```python
from build123d import *

# Parameters (mm, degrees)
BOSS_EXTRUDE1_DEPTH = 0.254
SKETCH2_R           = 4.699
CUT_EXTRUDE1_DEPTH  = 1.254
SKETCH3_W           = 2.54
SKETCH3_H           = 0.635
CUT_EXTRUDE2_DEPTH  = 1.254
SKETCH5_OUTSIDE_W   = 121.447
SKETCH5_OUTSIDE_H   = 109.618
CUT_EXTRUDE5_DEPTH  = 1.254


with BuildPart() as part:
    # Sketch1 → Boss-Extrude1 (new body)
    with BuildSketch(Plane.XY):
        with BuildLine():
            Line((67.21146711, 76.191723231), (8.696654013, 17.676910134))
            Line((8.696654013, 17.676910134), (7.228954972, 14.133571205))
            ThreePointArc((7.228954972, 14.133571205), (14.666587579, 6.075099489), (15.105587123, -4.88230096))
            Line((15.105587123, -4.88230096), (18.648926052, -6.35))
            Line((18.648926052, -6.35), (101.401368334, -6.35))
            ThreePointArc((101.401368334, -6.35), (93.866160503, 38.880636728), (67.21146711, 76.191723231))
        make_face()
        with BuildLine():
            Line((88.672924278, 6.35), (27.86051193, 6.35))
            ThreePointArc((27.86051193, 6.35), (26.399857642, 10.93517908), (24.190484974, 15.210228852))
            Line((24.190484974, 15.210228852), (67.191354125, 58.211098004))
            ThreePointArc((67.191354125, 58.211098004), (82.13289044, 34.020557137), (88.672924278, 6.35))
        make_face(mode=Mode.SUBTRACT)
    extrude(amount=BOSS_EXTRUDE1_DEPTH)

    # Sketch2 → Cut-Extrude1 (cut, through all)
    with BuildSketch(Plane.XY.offset(0.254)):
        with Locations((22.225, 0)):
            Circle(SKETCH2_R)
        with Locations((36.195, 0)):
            Circle(SKETCH2_R)
        with Locations((61.722, 0)):
            Circle(SKETCH2_R)
        with Locations((75.692, 0)):
            Circle(SKETCH2_R)
        with Locations((95.25, 0)):
            Circle(SKETCH2_R)
        with Locations((15.715448212, 15.715448212)):
            Circle(SKETCH2_R)
        with Locations((25.593729945, 25.593729945)):
            Circle(SKETCH2_R)
        with Locations((43.644044748, 43.644044748)):
            Circle(SKETCH2_R)
        with Locations((53.522326482, 53.522326482)):
            Circle(SKETCH2_R)
        with Locations((92.004434954, 24.652514046)):
            Circle(SKETCH2_R)
        with Locations((82.48891971, 47.625)):
            Circle(SKETCH2_R)
        with Locations((67.351920908, 67.351920908)):
            Circle(SKETCH2_R)
    extrude(amount=-CUT_EXTRUDE1_DEPTH, mode=Mode.SUBTRACT)

    # Sketch3 → Cut-Extrude2 (cut, through all)
    with BuildSketch(Plane.XY.offset(0.254)):
        Polygon((15.266435406, 24.246691527), (17.06248663, 26.042742751), (17.511499436, 25.593729945), (15.715448212, 23.797678721), align=None)
        Polygon((44.991083167, 53.971339288), (43.195031942, 52.175288063), (43.644044748, 51.726275257), (45.440095973, 53.522326482), align=None)
        with Locations((29.21, -6.0325)):
            Rectangle(SKETCH3_W, SKETCH3_H)
        with Locations((68.707, -6.0325)):
            Rectangle(SKETCH3_W, SKETCH3_H)
        Polygon((29.230733674, 38.210989795), (31.026784898, 40.007041019), (31.475797704, 39.558028213), (29.67974648, 37.761976989), align=None)
        Polygon((56.845021246, 65.825277367), (55.048970022, 64.029226143), (55.497982828, 63.580213337), (57.294034052, 65.376264561), align=None)
        with Locations((48.9585, -6.0325)):
            Rectangle(SKETCH3_W, SKETCH3_H)
        with Locations((85.471, -6.0325)):
            Rectangle(SKETCH3_W, SKETCH3_H)
        Polygon((99.935462164, 14.437711971), (100.266998693, 11.919442024), (101.526133667, 12.085210288), (101.194597138, 14.603480236), align=None)
        Polygon((93.765504959, 37.464305742), (94.938831965, 37.950313702), (93.966816047, 40.296967714), (92.793489041, 39.810959755), align=None)
        Polygon((79.327792988, 62.471156422), (80.874047017, 60.456038938), (81.88160576, 61.229165953), (80.33535173, 63.244283437), align=None)
        Polygon((13.593916116, 7.005422516), (14.565932035, 4.658768503), (15.739259041, 5.144776462), (14.767243123, 7.491430475), align=None)
    extrude(amount=-CUT_EXTRUDE2_DEPTH, mode=Mode.SUBTRACT)

    # Sketch5 outside → Cut-Extrude5 (cut, through all)
    with BuildSketch(Plane.XY.offset(0.254)):
        with Locations((54.4145, 34.921)):
            Rectangle(SKETCH5_OUTSIDE_W, SKETCH5_OUTSIDE_H)
        Polygon((53.971339288, 44.991083167), (64.029226143, 55.048970022), (55.048970022, 64.029226143), (44.991083167, 53.971339288), align=None, mode=Mode.SUBTRACT)
    extrude(amount=-CUT_EXTRUDE5_DEPTH, mode=Mode.SUBTRACT)


solid = part.part
```
Read the model definition and answer for the solid it produces. Units are mm, in the model's axes. Give positions to 0.01 mm unless a question says otherwise; leave off trailing zeros. Loops run counter-clockwise (first coordinate to the right, second up) from the corner with the lowest first, then second, coordinate; pieces in that order, holes last.
Item 1: The part is cut by section A-A (y = 56.25). Write down the section's boundary in (x, z).
Item 2: The part is cut by section D-D (y = 62). Write down the section's boundary in (x, z).
Item 3: The part is cut by section C-C (z = 0.1). Write down the section's boundary in (x, y).
Item 4: The part is cut by section B-B (x = 52.75). Write down the section's boundary in (y, z).
Item 5: Find the intervals of material crossed by line 1 along X through (y, z) = (50.25, 0.15); line 2 along Y through (x, z) = (55, 0.05); line 3 along X through (y, z) = (53, 0.2), in increasing order.
Taken from the geometry:
1. outline: (47.27, 0) - (49.7, 0) - (49.7, 0.25) - (47.27, 0.25) - close; (57.35, 0) - (62.83, 0) - (62.83, 0.25) - (57.35, 0.25) - close
2. outline: (53.02, 0) - (57.08, 0) - (57.08, 0.25) - (53.02, 0.25) - close
3. outline: (44.99, 53.97) - (53.97, 44.99) - (64.03, 55.05) - (55.05, 64.03) - close; hole circle Ø9.4 at (53.52, 53.52)
4. outline: (46.21, 0) - (48.89, 0) - (48.89, 0.25) - (46.21, 0.25) - close; (58.16, 0) - (61.73, 0) - (61.73, 0.25) - (58.16, 0.25) - close
5. line 1: x = 48.71 to 50.15, 56.89 to 59.23
5. line 2: y = 46.02 to 49.06, 57.98 to 63.98
5. line 3: x = 45.96 to 48.85, 58.19 to 61.98
